The drawing under review shows one solid part. Ordinate dimensions are in mm from its lowest x, y, z. Give positions to 0.01 mm unless a question says otherwise; leave off trailing zeros. Loops run counter-clockwise (first coordinate to the right, second up) from the corner with the lowest first, then second, coordinate; pieces in that order, holes last. Notation, with made-up numbers: (34.5, 73) -> (82.5, 73) arc R31 ccw to (82.5, 98) -> close; hole circle Ø3 at (43.5, 2.25). An arc over 180 degrees is marked (long way). Answer in a Markdown table with one row per item. Add a question column.
(1) For line 1 (X direction, y = 62.5, z = 103); line 2 (Y direction, x = 72, z = 26) (1 decimal); line 3 (Z direction, x = 7.5, y = 25), list the stretches that pass through material, from the lowest coordinate up.
(2) Consider section A-A on z = 14. Write out the cut boundary in (x, y), then the cut area to 3 significant figures.
(3) Consider section B-B on x = 10. Write out the cut boundary in (y, z).
(4) Consider section D-D on z = 103. Write out the cut boundary in (x, y).
(5) For pin 1 (8 mm diameter, centred on x = 30, y = 58, fed in from +Z), flat-tipped, find the tip position at first contact; note if it passes through.
(6) Draft analysis for pull direction X (two halves, no side actions). For the marked faces 1, 2 and 3, state which applies: +X half, -X half, draft (parallel to the pull), parting line (faces both ways), or undercut.
(7) Consider section C-C on y = 40.5. Write out the cut boundary in (x, z), then the cut area to 3 significant figures.
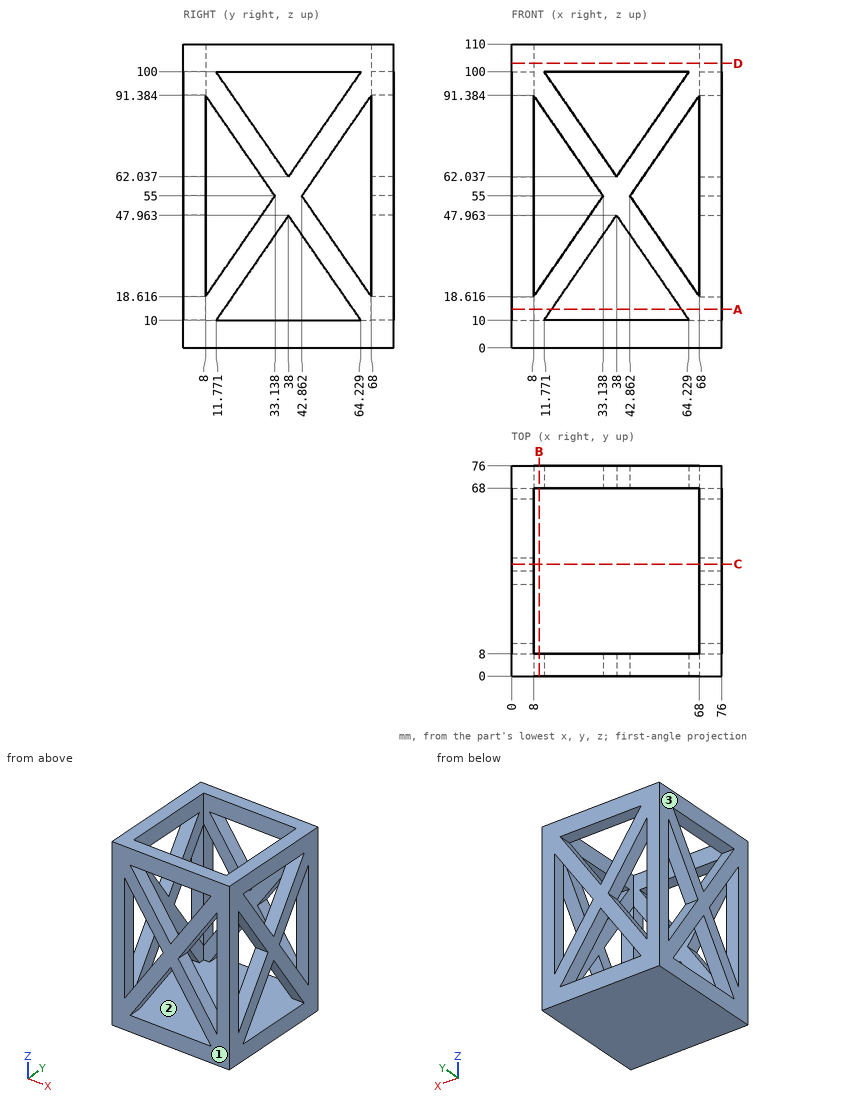
Values follow:
| question | item | result |
|---|---|---|
| 1 | line 1 | 0 to 8, 68 to 76 |
| 1 | line 2 | 0 to 8, 13.1 to 22.8, 53.2 to 62.9, 68 to 76 |
| 1 | line 3 | 0 to 10, 29.15 to 43.22, 66.78 to 80.85, 100 to 110 |
| 2 | outline | (0, 0) -> (14.53, 0) -> (14.53, 8) -> (8, 8) -> (8, 14.53) -> (0, 14.53) -> close; (0, 61.47) -> (8, 61.47) -> (8, 68) -> (14.53, 68) -> (14.53, 76) -> (0, 76) -> close; (61.47, 0) -> (76, 0) -> (76, 14.53) -> (68, 14.53) -> (68, 8) -> (61.47, 8) -> close; (61.47, 68) -> (68, 68) -> (68, 61.47) -> (76, 61.47) -> (76, 76) -> (61.47, 76) -> close |
| 2 | area | 674 mm2 |
| 3 | outline | (0, 0) -> (76, 0) -> (76, 21.51) -> (68, 21.51) -> (68, 10) -> (8, 10) -> (8, 21.51) -> (0, 21.51) -> close; (0, 88.49) -> (8, 88.49) -> (8, 110) -> (0, 110) -> close; (68, 88.49) -> (76, 88.49) -> (76, 110) -> (68, 110) -> close |
| 4 | outline | (0, 0) -> (76, 0) -> (76, 76) -> (0, 76) -> close; hole (8, 8) -> (68, 8) -> (68, 68) -> (8, 68) -> close |
| 5 | pin 1 | z = 10 |
| 6 | face 1 | draft |
| 6 | face 2 | undercut |
| 6 | face 3 | -X half |
| 7 | outline | (0, 0) -> (76, 0) -> (76, 10) -> (0, 10) -> close; (0, 44.34) -> (8, 44.34) -> (8, 65.66) -> (0, 65.66) -> close; (0, 100) -> (8, 100) -> (8, 110) -> (0, 110) -> close; (68, 44.34) -> (76, 44.34) -> (76, 65.66) -> (68, 65.66) -> close; (68, 100) -> (76, 100) -> (76, 110) -> (68, 110) -> close |
| 7 | area | 1,260 mm2 |
